from build123d import *

# Parameters (mm, degrees)
F0_W     = 100
F0_H     = 50
F1_DEPTH = 20
F2_R     = 10.225485
F3_DEPTH = 20.001
F4_W     = 24.237767
F4_H     = 12.803474
F5_DEPTH = 20.001
F6_W     = 19.731463
F6_H     = 7.589027
F7_DEPTH = 20


with BuildPart() as f1:
    # F0 (on Front) → F1 (new body)
    with BuildSketch(Plane.XZ):
        with Locations((50, 25)):
            Rectangle(F0_W, F0_H)
    extrude(amount=F1_DEPTH)

    # F2 (on Front) → F3 (cut, through all)
    with BuildSketch(Plane.XZ):
        with Locations((28.946707, 17.129513)):
            Circle(F2_R)
    extrude(amount=F3_DEPTH, mode=Mode.SUBTRACT)

    # F4 (on face) → F5 (cut, through all)
    with BuildSketch(Plane.XZ.offset(20)):
        with Locations((79.387456, 26.100426)):
            Rectangle(F4_W, F4_H)
    extrude(amount=-F5_DEPTH, mode=Mode.SUBTRACT)

    # F6 (on face) → F7 (join)
    with BuildSketch(Plane.XZ.offset(20)):
        with Locations((21.223658, 39.137683)):
            Rectangle(F6_W, F6_H)
    extrude(amount=F7_DEPTH)


solid = f1.part
The model under review builds one solid part; all positions refer to its coordinate system, in mm. A direction names the side the tool comes from. Coordinates: 2 decimals unless noted, no trailing zeros. Loops run counter-clockwise (first coordinate to the right, second up) from the corner with the lowest first, then second, coordinate; pieces in that order, holes last. Notation, with made-up numbers: M -7.5,76.25 L 32.5,76.25 A17 cw 32.5,86.25 Z; hole C 22,67 d9. An arc over 180 degrees is marked long. Put each result on its own line as item: value. Start each with the question number.
Q1. Wall thickness on line 1 (Z direction, x = 79, y = -19.5); line 2 (X direction, y = -15, z = 24); line 3 (Y direction, x = 14, z = 7.5): over which ranges is each line inside the solid? List them lowest first.
Q2. Clearance check with flat-ended pins moving along their axes: pin 1 (8.5 mm diameter, centred on y = -27, z = 38, fed in from -X); pin 2 (6 mm diameter, centred on y = -26.5, z = 40, fed in from +X); pin 3 (10 mm diameter, centred on x = 16.5, y = -34, fed in from -Z). State where each tip first meets the part, or that it passes through.
Q3. Add section D-D (y = -12.5). Write out the cut boundary in (x, z), and give its area (3 significant figures).
Q4. Add section C-C (z = 37.5). Write out the cut boundary in (x, y), and give its area (3 significant figures).
Q5. For faces 1 (the flat face through (21, -30, 35.343)), 2 (the flat face through (11.358, -30, 39)), 3 (the flat face through (21, -30, 42.932)), 4 (the flat face through (91.506, -10, 26)), list the 3-axis set-ups (+Z, -Z, +X, -X, +Y, -Y) from which the entire face can be reached by the end or side of a thin tool; tool diameter is ignored.
Q6. Add section B-B (z = 21). Write out the cut boundary in (x, y), and give its area (3 significant figures).
Q7. The part is to be moulded in two halves that separate along Z. For faces 5 (the flat face through (79, -10, 32.502)), 6 (the flat face through (31.089, -30, 39)), 7 (the flat face through (49, -10, 0)), say which applies: +Z half, -Z half, draft (parallel to the pull), parting line (faces both ways), or undercut.
Q8. Add section A-A (x = 87). Write out the cut boundary in (y, z), and give its area (3 significant figures).
Answers:
1. line 1: z = 0 to 19.7, 32.5 to 50
1. line 2: x = 0 to 21.37, 36.52 to 67.27, 91.51 to 100
1. line 3: y = -20 to 0
2. pin 1: stops at x = 11.36
2. pin 2: stops at x = 31.09
2. pin 3: stops at z = 35.34
3. outline: M 0,0 L 100,0 L 100,50 L 0,50 Z; hole C 28.95,17.13 d20.45; hole M 67.27,19.7 L 91.51,19.7 L 91.51,32.5 L 67.27,32.5 Z
3. area: 4,360 mm^2
4. outline: M 0,-20 L 11.36,-20 L 11.36,-40 L 31.09,-40 L 31.09,-20 L 100,-20 L 100,0 L 0,0 Z
4. area: 2,390 mm^2
5. face 1: -Z, +X, -X, -Y
5. face 2: +Z, -Z, -X, -Y
5. face 3: +Z, +X, -X, -Y
5. face 4: +Y, -Y
6. outline: M 0,-20 L 19.48,-20 L 19.48,0 L 0,0 Z; M 38.41,-20 L 67.27,-20 L 67.27,0 L 38.41,0 Z; M 91.51,-20 L 100,-20 L 100,0 L 91.51,0 Z
6. area: 1,140 mm^2
7. face 5: undercut
7. face 6: draft
7. face 7: -Z half
8. outline: M -20,0 L 0,0 L 0,19.7 L -20,19.7 Z; M -20,32.5 L 0,32.5 L 0,50 L -20,50 Z
8. area: 744 mm^2
